Part model, mm, in its own coordinate system. Face numbers are marked on the shaded views. A direction names the side the tool comes from. Give positions to 0.01 mm unless a question says otherwise; leave off trailing zeros. Order: outer loops, then holes, each group sorted by start corner. A loop starts at its lowest first (then second) coordinate and runs counter-clockwise, first axis right, second up. Notation, with made-up numbers: M 26.25,46.25 L 30.25,46.25 A27 ccw 30.25,69.25 Z; hole C 40.5,6 d6. An arc over 180 degrees is marked long. Answer as a JSON object with one key per item and string values.
from build123d import *

# Parameters (mm, degrees)
BOSS_EXTRUDE1_DEPTH      = 5.08
BOSS_EXTRUDE2_DEPTH      = 154.427309
BOSS_EXTRUDE2_DEPTH_BACK = 154.427309
SKETCH2_R                = 2.54
SKETCH2_W                = 2.54
SKETCH2_H                = 5.08
SKETCH3_W                = 12.7
SKETCH3_H                = 6.227195603
CUT_EXTRUDE1_DEPTH       = 5.08
BOSS_EXTRUDE3_DEPTH      = 39.37
SKETCH5_W                = 138.751749018
SKETCH5_H                = 37.67744757
CUT_EXTRUDE2_DEPTH       = 5.08
SKETCH6_W                = 11.329576632
SKETCH6_H                = 15.748
BOSS_EXTRUDE4_DEPTH      = 99.568
SKETCH7_W                = 58.494788807
SKETCH7_H                = 56.964758344
CUT_EXTRUDE3_DEPTH       = 5.08
LIP1_START               = -12.594044208
LIP1_DEPTH               = 99.568
LIP2_START               = -12.594044208
LIP2_DEPTH               = 99.568
CUT_EXTRUDE4_REACH       = 261.821
SKETCH8_R                = 1.55


# Read off the part's stored shape, not the designer's step: Lip1, Lip2
with BuildPart() as part:
    # Sketch1 → Boss-Extrude1 (new body)
    with BuildSketch(Plane(origin=(0, 0, 0), x_dir=(1, 0, 0), z_dir=(0, 1, 0))):
        with BuildLine():
            ThreePointArc((-150.649044256, 36.211449361), (-152.994577449, 24.475760888), (-154.427308629, 12.594044208))
            Line((-154.427308629, 12.594044208), (0, 12.594044208))
            Line((0, 12.594044208), (0, 106.558758971))
            Line((0, 106.558758971), (-63.290413745, 106.558758971))
            ThreePointArc((-63.290413745, 106.558758971), (-92.01449877, 83.028775744), (-112.479484736, 52.046240008))
            Line((-112.479484736, 52.046240008), (-150.649044256, 36.211449361))
        make_face()
        with BuildLine():
            Line((0, 106.558758971), (0, 12.594044208))
            Line((0, 12.594044208), (154.427308629, 12.594044208))
            ThreePointArc((154.427308629, 12.594044208), (152.994577449, 24.475760888), (150.649044256, 36.211449361))
            Line((150.649044256, 36.211449361), (112.479484736, 52.046240008))
            ThreePointArc((112.479484736, 52.046240008), (92.01449877, 83.028775744), (63.290413745, 106.558758971))
            Line((63.290413745, 106.558758971), (0, 106.558758971))
        make_face()
    extrude(amount=BOSS_EXTRUDE1_DEPTH)

    # Sketch2 → Boss-Extrude2 (add, two sides: drawn at the far end of the back side and taken through both)
    with BuildSketch(Plane(origin=(0, 0, 0), x_dir=(0, 0, -1), z_dir=(1, 0, 0)).offset(-BOSS_EXTRUDE2_DEPTH_BACK)):
        with Locations((10.054044208, 2.54)):
            Circle(SKETCH2_R)
        with Locations((11.324044208, 2.54)):
            Rectangle(SKETCH2_W, SKETCH2_H)
    extrude(amount=BOSS_EXTRUDE2_DEPTH + BOSS_EXTRUDE2_DEPTH_BACK)

    # Sketch3 → Cut-Extrude1 (cut)
    with BuildSketch(Plane(origin=(0, 5.08, 0), x_dir=(1, 0, 0), z_dir=(0, 1, 0))):
        with Locations((-116.835308629, 9.480446407)):
            Rectangle(SKETCH3_W, SKETCH3_H)
        with Locations((-148.077308629, 9.480446407)):
            Rectangle(SKETCH3_W, SKETCH3_H)
        with Locations((-85.593308629, 9.480446407)):
            Rectangle(SKETCH3_W, SKETCH3_H)
        with Locations((-54.351308629, 9.480446407)):
            Rectangle(SKETCH3_W, SKETCH3_H)
        with Locations((-23.109308629, 9.480446407)):
            Rectangle(SKETCH3_W, SKETCH3_H)
        with Locations((8.132691371, 9.480446407)):
            Rectangle(SKETCH3_W, SKETCH3_H)
        with Locations((39.374691371, 9.480446407)):
            Rectangle(SKETCH3_W, SKETCH3_H)
        with Locations((70.616691371, 9.480446407)):
            Rectangle(SKETCH3_W, SKETCH3_H)
        with Locations((101.858691371, 9.480446407)):
            Rectangle(SKETCH3_W, SKETCH3_H)
        with Locations((133.100691371, 9.480446407)):
            Rectangle(SKETCH3_W, SKETCH3_H)
    extrude(amount=-CUT_EXTRUDE1_DEPTH, mode=Mode.SUBTRACT)

    # Sketch4 → Boss-Extrude3 (add)
    with BuildSketch(Plane.XZ):
        with BuildLine():
            Line((-53.354740134, -106.481309786), (-53.354740134, -91.517526844))
            ThreePointArc((-53.354740134, -91.517526844), (-82.728496733, -66.340222196), (-101.149908104, -32.320142108))
            Line((-101.149908104, -32.320142108), (-101.149908104, -52.046240008))
            Line((-101.149908104, -52.046240008), (-112.479484736, -52.046240008))
            Line((-112.479484736, -52.046240008), (-100.285956923, -61.644665115))
            ThreePointArc((-100.285956923, -61.644665115), (-80.038963099, -87.43196163), (-53.354740134, -106.481309786))
        make_face()
        Polygon((-101.149908104, -52.046240008), (-101.149908104, -32.320142108), (-101.149908104, -12.594044208), (-110.485308629, -12.594044208), (-112.479484736, -12.594044208), (-112.479484736, -52.046240008), align=None)
        with BuildLine():
            Line((99.574939951, -61.644665115), (112.479484736, -52.046240008))
            Line((112.479484736, -52.046240008), (101.149908104, -52.046240008))
            Line((101.149908104, -52.046240008), (101.149908104, -32.320142108))
            ThreePointArc((101.149908104, -32.320142108), (82.470268628, -66.658795409), (52.643723162, -91.92634826))
            Line((52.643723162, -91.92634826), (52.643723162, -106.481309786))
            ThreePointArc((52.643723162, -106.481309786), (79.327946127, -87.43196163), (99.574939951, -61.644665115))
        make_face()
        Polygon((112.479484736, -52.046240008), (112.479484736, -12.594044208), (108.208691371, -12.594044208), (101.149908104, -12.594044208), (101.149908104, -32.320142108), (101.149908104, -52.046240008), align=None)
    extrude(amount=BOSS_EXTRUDE3_DEPTH)

    # Sketch5 → Cut-Extrude2 (cut)
    with BuildSketch(Plane.XZ):
        with Locations((0, -42.458273938)):
            Rectangle(SKETCH5_W, SKETCH5_H)
    extrude(amount=-CUT_EXTRUDE2_DEPTH, mode=Mode.SUBTRACT)

    # Sketch6 → Boss-Extrude4 (add)
    with BuildSketch(Plane.XY.offset(-12.594044208)):
        with Locations((-106.81469642, -31.496)):
            Rectangle(SKETCH6_W, SKETCH6_H)
        with Locations((106.81469642, -31.496)):
            Rectangle(SKETCH6_W, SKETCH6_H)
    extrude(amount=BOSS_EXTRUDE4_DEPTH)

    # Sketch7 → Cut-Extrude3 (cut)
    with BuildSketch(Plane(origin=(0, 5.08, 0), x_dir=(1, 0, 0), z_dir=(0, 1, 0))):
        with Locations((-146.082703033, 21.756830304)):
            Rectangle(SKETCH7_W, SKETCH7_H)
        with Locations((146.082703033, 21.756830304)):
            Rectangle(SKETCH7_W, SKETCH7_H)
    extrude(amount=-CUT_EXTRUDE3_DEPTH, mode=Mode.SUBTRACT)

    # Lip1 outline → Lip1 (add)
    with BuildSketch(Plane.XY.offset(LIP1_START)):
        Polygon((-112.479484736, -23.622), (-114.511484736, -23.622), (-114.511484736, -25.730085067), (-112.479484736, -26.162), align=None)
    extrude(amount=LIP1_DEPTH)

    # Lip2 outline → Lip2 (add)
    with BuildSketch(Plane.XY.offset(LIP2_START)):
        Polygon((114.511484736, -23.622), (112.479484736, -23.622), (112.479484736, -26.162), (114.511484736, -25.730085067), align=None)
    extrude(amount=LIP2_DEPTH)

    # Cut-Extrude4: up to this face of the body (flat: up to its plane)
    cut_extrude4_end = Plane(part.part.faces().sort_by_distance((-116.835308629, 2.54, -31.416626842))[0])
    # Sketch8 → Cut-Extrude4 (cut, up to the picked face)
    with BuildSketch(Plane(origin=(116.835308629, 0, 0), x_dir=(0, 0, -1), z_dir=(1, 0, 0)), mode=Mode.PRIVATE) as cut_extrude4_sk1:
        with Locations((10.054044208, 2.54)):
            Circle(SKETCH8_R)
    cut_extrude4_tool1 = split(extrude(cut_extrude4_sk1.sketch, amount=-CUT_EXTRUDE4_REACH, mode=Mode.PRIVATE), bisect_by=cut_extrude4_end, keep=Keep.BOTH, mode=Mode.PRIVATE)
    add(cut_extrude4_tool1.solids().sort_by(Axis((116.835309, 2.54, -10.054044), (-1, 0, 0)))[0], mode=Mode.SUBTRACT)


solid = part.part
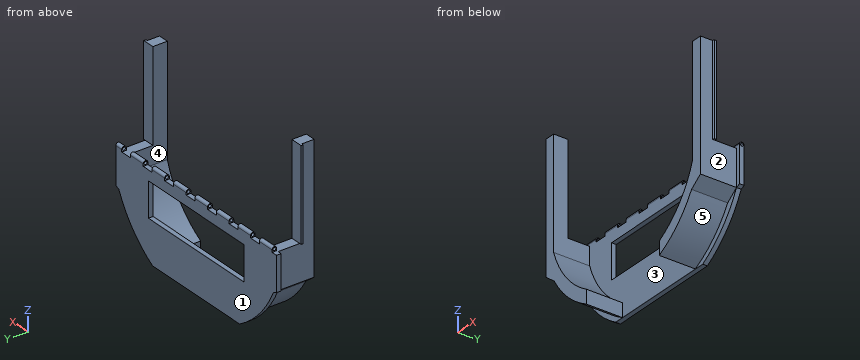
1. Probe line 1 along X through (y, z) = (-33.5, -13); line 2 along X through (y, z) = (-33, -34); line 3 along Y through (x, z) = (0, -13.5). List the from-to ranges inside material, lowest first.
Worked answers:
{"line 1": "x = -112.48 to -101.15, 101.15 to 112.48", "line 2": "x = -112.48 to -100.59, 100.59 to 112.48", "line 3": "y = 0 to 5.08"}
2. Cut at D-D on z = -26.5. Give the cut face in (x, y).
Worked answers:
{"outline": "M -116.84,0 L -112.48,0 L -112.48,-39.37 L -101.15,-39.37 L -101.15,0 L -69.38,0 L -69.38,5.08 L -116.84,5.08 Z; M 69.38,0 L 101.15,0 L 101.15,-39.37 L 112.48,-39.37 L 112.48,0 L 116.84,0 L 116.84,5.08 L 69.38,5.08 Z"}
3. Cut at C-C on y = -4.5. Give the cut face in (x, z).
Worked answers:
{"outline": "M -112.48,-52.05 L -100.29,-61.64 A115.35 ccw -53.35,-106.48 L -53.35,-91.52 A106.33 cw -101.15,-32.32 L -101.15,-12.59 L -112.48,-12.59 Z; M 52.64,-106.48 A115.35 ccw 99.57,-61.64 L 112.48,-52.05 L 112.48,-12.59 L 101.15,-12.59 L 101.15,-32.32 A106.33 cw 52.64,-91.93 Z"}
4. Cut at A-A on x = 21.5. Give the cut face in (y, z).
Worked answers:
{"outline": "M 0,-106.56 L 5.08,-106.56 L 5.08,-61.3 L 0,-61.3 Z; M 0,-23.62 L 5.08,-23.62 L 5.08,-10.05 A2.54 ccw 0,-10.05 Z; hole C 2.54,-10.05 d3.1"}
5. Two-plate mould, pull along X, no slides. Class the marked faces 1, 2 and 3: +X half, -X half, draft (parallel to the pull), parting line (faces both ways), or undercut.
Worked answers:
{"face 1": "draft", "face 2": "+X half", "face 3": "undercut"}
6. Which spindle directions (+Z, -Z, +X, -X, +Y, -Y) get a long thin tool onto all of the face, cutting with end or side? Do the marked faces 4 and 5. Say none if no direction does.
Worked answers:
{"face 4": "+Z, -Y", "face 5": "-Z, +X, -Y"}
7. Pin check, flat tips, straight feed: P1, Ø1, axis at y = -14.5, z = -83.5, coming from the +X side; P2, Ø5, axis at y = 2.54, z = -10.05, coming from the -X side; P3, Ø2.5, axis at y = 3, z = -11.5, coming from the -X side; P4, Ø4, axis at x = -24, y = 3, coming from the +Z side. Stop position of each tip, or through.
Worked answers:
{"P1": "stops at x = 83.72", "P2": "stops at x = -110.49", "P3": "stops at x = -116.84", "P4": "stops at z = -12.59"}
8. Cut at B-B on z = 3. Give the cut face in (x, y), plus the area to 3 significant figures.
Worked answers:
{"outline": "M -114.51,-25.73 L -112.48,-26.16 L -112.48,-39.37 L -101.15,-39.37 L -101.15,-23.62 L -114.51,-23.62 Z; M 101.15,-39.37 L 112.48,-39.37 L 112.48,-26.16 L 114.51,-25.73 L 114.51,-23.62 L 101.15,-23.62 Z", "area": "366 mm^2"}
